Autodesk Fusion 360 part; units mm, degrees
sketch "Sketch1" plane through (0, 0, 0) normal (0, 1, 0) x (1, 0, 0)
  line L0 (0, 0) -> (88.9, 0)
  line L1 (88.9, 0) -> (88.9, -109.22)
  line L2 (88.9, -109.22) -> (0, -109.22)
  line L3 (0, -109.22) -> (0, 0)
  dimension "d1" = 88.9
  dimension "d2" = 109.22
extrude "Extrude1" add sketch "Sketch1" along normal blind 6.35
fillet "Fillet1" radius 7.62 4 edges at (88.9, 3.175, 0) (0, 3.175, 0) (88.9, 3.175, 109.22) (0, 3.175, 109.22)
sketch "Sketch2" plane through (0, 6.35, 0) normal (0, 1, 0) x (-1, 0, 0)
  arc A0 (0, 101.6) -> (-7.62, 109.22) centre (-7.62, 101.6) ccw
  line L0 (-7.62, 109.22) -> (-81.28, 109.22)
  arc A1 (-81.28, 109.22) -> (-88.9, 101.6) centre (-81.28, 101.6) ccw
  line L1 (-88.9, 101.6) -> (-88.9, 7.62)
  arc A2 (-88.9, 7.62) -> (-81.28, 0) centre (-81.28, 7.62) ccw
  line L2 (-81.28, 0) -> (-7.62, 0)
  arc A3 (-7.62, 0) -> (0, 7.62) centre (-7.62, 7.62) ccw
  line L3 (0, 7.62) -> (0, 101.6)
  line L4 (-63.8008, 109.22) -> (-63.8008, 101.6)
  line L5 (-88.9, 94.0515) -> (-81.28, 94.0515)
  line L6 (-81.28, 101.6) -> (-7.62, 101.6)
  line L7 (-7.62, 101.6) -> (-7.62, 7.62)
  line L8 (-7.62, 7.62) -> (-81.28, 7.62)
  line L9 (-81.28, 7.62) -> (-81.28, 101.6)
  line L10 (-7.62, 7.62) -> (-5.08, 5.08)
hole "Hole1" at (5.08, 6.35, 5.08) direction (0, -1, 0) diameter 3.175 end through all
sketch "Sketch3" plane through (0, 6.35, 0) normal (0, 1, 0) x (-1, 0, 0)
  circle A0 centre (-5.08, 5.08) radius 1.5875
  arc A1 (0, 101.6) -> (-7.62, 109.22) centre (-7.62, 101.6) ccw
  line L0 (-7.62, 109.22) -> (-81.28, 109.22)
  arc A2 (-81.28, 109.22) -> (-88.9, 101.6) centre (-81.28, 101.6) ccw
  line L1 (-88.9, 101.6) -> (-88.9, 7.62)
  arc A3 (-88.9, 7.62) -> (-81.28, 0) centre (-81.28, 7.62) ccw
  line L2 (-81.28, 0) -> (-7.62, 0)
  arc A4 (-7.62, 0) -> (0, 7.62) centre (-7.62, 7.62) ccw
  line L3 (0, 7.62) -> (0, 101.6)
  line L4 (-50.8, 0) -> (-50.8, 7.62)
  line L5 (-88.9, 22.8139) -> (-81.28, 22.8139)
  line L6 (-81.28, 7.62) -> (-7.62, 7.62)
  line L7 (-7.62, 7.62) -> (-7.62, 101.6)
  line L8 (-7.62, 101.6) -> (-81.28, 101.6)
  line L9 (-81.28, 101.6) -> (-81.28, 7.62)
  line L10 (-81.28, 7.62) -> (-83.82, 5.08)
  line L11 (-7.62, 101.6) -> (-5.08, 104.14)
  line L12 (-81.28, 101.6) -> (-83.82, 104.14)
hole "Hole2" at (83.82, 6.35, 5.08) direction (0, -1, 0) diameter 3.175 end through all
sketch "Sketch4" plane through (0, 6.35, 0) normal (0, 1, 0) x (-1, 0, 0)
  circle A0 centre (-83.82, 5.08) radius 1.5875
  circle A1 centre (-5.08, 5.08) radius 1.5875
  arc A2 (0, 101.6) -> (-7.62, 109.22) centre (-7.62, 101.6) ccw
  line L0 (-7.62, 109.22) -> (-81.28, 109.22)
  arc A3 (-81.28, 109.22) -> (-88.9, 101.6) centre (-81.28, 101.6) ccw
  line L1 (-88.9, 101.6) -> (-88.9, 7.62)
  arc A4 (-88.9, 7.62) -> (-81.28, 0) centre (-81.28, 7.62) ccw
  line L2 (-81.28, 0) -> (-7.62, 0)
  arc A5 (-7.62, 0) -> (0, 7.62) centre (-7.62, 7.62) ccw
  line L3 (0, 7.62) -> (0, 101.6)
  line L4 (0, 73.66) -> (-7.62, 73.66)
  line L5 (-28.8405, 109.22) -> (-28.8405, 101.6)
  line L6 (-7.62, 101.6) -> (-81.28, 101.6)
  line L7 (-81.28, 101.6) -> (-81.28, 60.96)
  line L8 (-81.28, 60.96) -> (-7.62, 60.96)
  line L9 (-7.62, 60.96) -> (-7.62, 101.6)
  line L10 (-44.45, 60.96) -> (-44.45, 101.6)
  line L11 (-7.62, 101.6) -> (-5.08, 104.14)
  line L12 (-81.28, 101.6) -> (-83.82, 104.14)
  point P0 (-83.82, 104.14)
  point P1 (-5.08, 104.14)
hole "Hole3" at (5.08, 6.35, 104.14) at (83.82, 6.35, 104.14) direction (0, -1, 0) diameter 3.175 end through all
thread "Thread1"
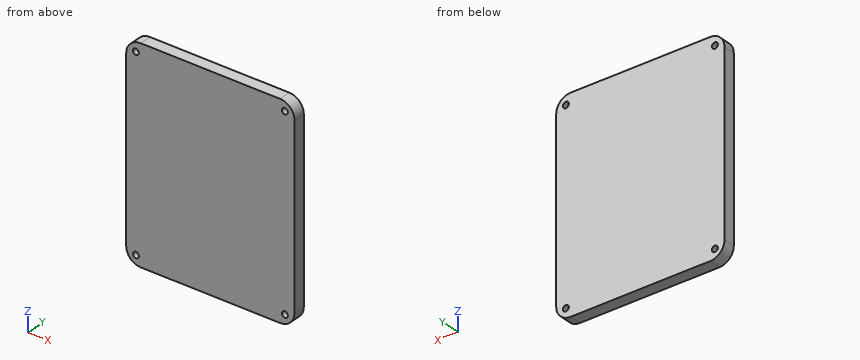
Geometry: final body of the model. Coordinates: model frame, mm. Coordinates: 2 decimals unless noted, no trailing zeros. Write each loop counter-clockwise with the first axis right and the second up, starting at its lowest first coordinate (ties: lowest second). Pieces come first, ordered by that corner, then holes. Notation, with made-up numbers: M 76.25,17 L 124.25,17 A23 cw 124.25,42 Z; hole C -19,-33 d10. An arc over 180 degrees is marked long. Use CSV: the item, a comma, the result in double quotes. Start each with the question number.
1. Cut plane A-A on x = 83.82. Return the cut outline in (y, z), plus the area to 3 significant figures.
2. Cut plane B-B on z = 104.14. Return the cut outline in (x, y), plus the area to 3 significant figures.
3. Ray query, probe 1 along X at (y, z) = (4.5, 5.08); probe 2 along Z at (x, y) = (5.08, 4); probe 3 along X at (y, z) = (3.75, 103). Return the intervals inside material, ascending.
4. First-contact query: P1, Ø3, axis at x = 5.08, z = 5.08, coming from the -Y side. Flat tip, straight axial feed; report the tip coordinate or a pass-through.
Entries:
1,outline,"M 0,0.44 L 6.35,0.44 L 6.35,3.49 L 0,3.49 Z; M 0,6.67 L 6.35,6.67 L 6.35,102.55 L 0,102.55 Z; M 0,105.73 L 6.35,105.73 L 6.35,108.78 L 0,108.78 Z"
1,area,"648 mm²"
2,outline,"M 0.44,0 L 3.49,0 L 3.49,6.35 L 0.44,6.35 Z; M 6.67,0 L 82.23,0 L 82.23,6.35 L 6.67,6.35 Z; M 85.41,0 L 88.46,0 L 88.46,6.35 L 85.41,6.35 Z"
2,area,"519 mm²"
3,probe 1,"0.44 to 3.49, 6.67 to 82.23, 85.41 to 88.46"
3,probe 2,"0.44 to 3.49, 6.67 to 102.55, 105.73 to 108.78"
3,probe 3,"0.13 to 3.98, 6.18 to 82.72, 84.92 to 88.77"
4,P1,"through"
